```python
from build123d import *

# Parameters (mm, degrees)
FILLET4_R     = 0.127
FILLET1_R     = 0.5
FILLET2_R     = 2
CHAMFER4_SIZE = 0.508


with BuildPart() as part:
    # Sketch1 → Revolve1 (revolve)
    with BuildSketch(Plane.XY, mode=Mode.PRIVATE) as revolve1_sk:
        Polygon((-10.16, 0), (-12.7, 0), (-12.7, 1.5875), (-11.4681, 1.5875), (-11.4681, 2.7559), (-12.7, 2.7559), (-12.7, 12.2809), (-15.0114, 12.2809), (-15.0114, 14.8209), (-13.0175, 14.8209), (-13.0175, 18.3769), (-15.0114, 18.3769), (-15.0114, 24.9809), (-10.16, 24.9809), (0, 24.9809), (0, 0), align=None)
    revolve(revolve1_sk.sketch.rotate(Axis((0, 0, 0), (0, 1, 0)), 270), axis=Axis((0, 0, 0), (0, 1, 0)))

    # Fillet4
    fillet4_edges = [part.edges().sort_by_distance(p)[0] for p in [
        (0, 18.3769, 13.0175),
        (0, 14.8209, 13.0175),
    ]]
    fillet(fillet4_edges, radius=FILLET4_R)

    # Sketch9 → Cut-Revolve2 (revolve, cut)
    with BuildSketch(Plane.XY, mode=Mode.PRIVATE) as cut_revolve2_sk:
        Polygon((10.25, 0), (9.499743762, 2.7999944), (9.499743762, 4.0699944), (10, 4.0699944), (10, 5.1699944), (9.525, 5.1699944), (9.525, 10.5039944), (0.396875, 10.5039944), (0.396875, 24.9809), (0, 24.9809), (0, 0), align=None)
    revolve(cut_revolve2_sk.sketch.rotate(Axis((0, 0, 0), (0, 1, 0)), 90), axis=Axis((0, 0, 0), (0, 1, 0)), mode=Mode.SUBTRACT)

    # Fillet1
    # the kernel refuses this fillet: 0.5 mm, written as the material it takes off along each edge
    with BuildSketch(Plane(origin=(0, 0, 0), x_dir=(0, 0, -1), z_dir=(1, 0, 0))) as fillet1_piece_1:
        with BuildLine():
            CenterArc((10.25 + FILLET1_R * 0.767326987979, FILLET1_R), FILLET1_R, 195, 75)
            Line((10.25 - FILLET1_R * 0.19859883831, FILLET1_R * 0.741180954897), (10.25, 0))
            Line((10.25, 0), (10.25 + FILLET1_R * 0.767326987979, 0))
        make_face()
    revolve(axis=Axis((0, 0, 0), (0, 1, 0)), mode=Mode.SUBTRACT)
    with BuildSketch(Plane(origin=(0, 5.1699944, 0), x_dir=(0, 0, -1), z_dir=(1, 0, 0))) as fillet1_piece_2_section:
        with BuildLine():
            CenterArc((9.525 + FILLET1_R, FILLET1_R), FILLET1_R, 180, 90)
            Line((9.525 + FILLET1_R, 0), (9.525, 0))
            Line((9.525, 0), (9.525, FILLET1_R))
        make_face()
    fillet1_piece_2 = revolve(axis=Axis((0, 5.1699944, 0), (0, 1, 0)), mode=Mode.PRIVATE)
    fillet1_piece_2 = fillet1_piece_2 & Plane(origin=(0, 5.314596345, 0), x_dir=(0, 0, -1), z_dir=(0, 1, 0)) * Cylinder(10, 41, mode=Mode.PRIVATE)
    add(fillet1_piece_2, mode=Mode.SUBTRACT)

    # Fillet2
    fillet2_edges = [part.edges().sort_by_distance(p)[0] for p in [
        (0, 2.7999944, 9.499743762),
    ]]
    fillet(fillet2_edges, radius=FILLET2_R)

    # Sketch11 → Upchurch Cone Fitting (revolve, cut)
    with BuildSketch(Plane.XY, mode=Mode.PRIVATE) as upchurch_cone_fitting_sk:
        Polygon((0.508, 14.5669), (0.508, 10.5039944), (0, 10.5039944), (0, 24.9809), (2.08066419, 24.9809), (2.08066419, 18.6817), (1.6002, 18.39300799), (0.8509, 16.334323159), (0.8509, 14.5669), align=None)
    revolve(upchurch_cone_fitting_sk.sketch.rotate(Axis((0, 0, 0), (0, 1, 0)), 90), axis=Axis((0, 0, 0), (0, 1, 0)), mode=Mode.SUBTRACT)

    # Chamfer4
    chamfer4_edges = [part.edges().sort_by_distance(p)[0] for p in [
        (0, 24.9809, 2.08066419),
    ]]
    chamfer(chamfer4_edges, length=CHAMFER4_SIZE)


solid = part.part
```
Here's how the part is built. I have some questions about the finished solid (model axes, mm). A direction names the side the tool comes from. Coordinates: 2 decimals unless noted, no trailing zeros. Write each loop counter-clockwise with the first axis right and the second up, starting at its lowest first coordinate (ties: lowest second). Pieces come first, ordered by that corner, then holes. Notation, with made-up numbers: (84.5, -21) -> (100.5, -21) arc R19 cw to (100.5, 1) -> close; hole circle Ø3 at (-13, 28.25). An arc over 180 degrees is marked (long way). Use a Markdown table: item, result. Add a question column.
(1) Please list where these lines run through material, in increasing order: line 1 (Y direction, x = -3, z = 11.5); line 2 (X direction, y = 4.4, z = 0); line 3 (Z direction, x = -1.5, y = 20.5).
(2) I'm going to push flat-ended pins straight in: P1, Ø5, axis at x = 0, z = 0, coming from the -Y side; P2, Ø0.9, axis at x = 0, z = 0, coming from the +Y side (3 decimals); P3, Ø5, axis at x = -5.5, y = 18.5, coming from the +Z side; P4, Ø6, axis at y = 17.5, z = -9.5, coming from the -X side. Where does each tip first touch, or does it pass through?
(3) For faces 1 (the cylindrical face through (9.76, 4.63, 2.17)), 2 (the cylindrical face through (-1.41, 21.54, 1.53)), 3 (the cylindrical face through (3.638, 3.574, -8.775)), 4 (the cylindrical face through (0.5, 12.5, 0.1)), which set-ups out of +Z, -Z, +X, -X, +Y, -Y let a thin tool reach every point of the face, with its end or its side?
(4) We'd pull the mould along Y, two halves only. Please class faces 5 (the conical face through (0.93, 16.89, -0.49)), 6 (the cylindrical face through (-9.67, 2.18, -6.165)), 7 (the flat face through (-7, 12.281, -11)): +Y half, -Y half, draft (parallel to the pull), parting line (faces both ways), or undercut.
(5) If we section it at A-A, the plane y = 22.5: Write out the boundary of the cut face in (x, z), and give its area (3 significant figures).
(6) If we section it at B-B, the plane y = 11.75: Write out the boundary of the cut face in (x, z), and give its area (3 significant figures).
Outcome:
| question | item | result |
|---|---|---|
| 1 | line 1 | y = 0 to 1.59, 2.76 to 24.98 |
| 1 | line 2 | x = -12.7 to -10, 10 to 12.7 |
| 1 | line 3 | z = -14.94 to -1.44, 1.44 to 14.94 |
| 2 | P1 | stops at y = 10.5 |
| 2 | P2 | passes through |
| 2 | P3 | stops at z = 14.71 |
| 2 | P4 | stops at x = -13.47 |
| 3 | face 1 | none |
| 3 | face 2 | +Y |
| 3 | face 3 | -Y |
| 3 | face 4 | +Y, -Y |
| 4 | face 5 | +Y half |
| 4 | face 6 | undercut |
| 4 | face 7 | -Y half |
| 5 | outline | circle Ø30.02 at (0, 0); hole circle Ø4.16 at (0, 0) |
| 5 | area | 694 mm^2 |
| 6 | outline | circle Ø25.4 at (0, 0); hole circle Ø1.02 at (0, 0) |
| 6 | area | 506 mm^2 |
